from build123d import *

# Parameters (mm, degrees)
BOSS_EXTRUDE1_DEPTH   = 160
RIB3_REACH            = 111.505
SKETCH4_WALL_W        = 239.367706636
SKETCH4_WALL_H        = 3
RIB4_START            = -3
RIB4_DEPTH            = 3
F_6_CLEARANCE_HOLE1_D = 3.7973
SKETCH18_R            = 2.3495
CUT_EXTRUDE1_DEPTH    = 7.5
SKETCH19_R            = 2.6162
CUT_EXTRUDE2_DEPTH    = 6.35
SKETCH10_R            = 2.3495
CUT_EXTRUDE3_DEPTH    = 163.255727865
SKETCH20_R            = 2.6162
CUT_EXTRUDE4_DEPTH    = 6.35


# Read off the part's stored shape, not the designer's step: Rib4
with BuildPart() as part:
    # Sketch1 → Boss-Extrude1 (new body)
    with BuildSketch(Plane.XY):
        with BuildLine():
            Line((0, 0), (0, 12))
            Line((0, 12), (-8, 12))
            Line((-8, 12), (-8, 6))
            ThreePointArc((-8, 6), (-8.878679656, 3.878679656), (-11, 3))
            Line((-11, 3), (-24, 3))
            Line((-24, 3), (-24, 0))
            Line((-24, 0), (-8.5, 0))
            Line((-8.5, 0), (-8.5, -0.285))
            Line((-8.5, -0.285), (0, -0.285))
            Line((0, -0.285), (0, 0))
        make_face()
    extrude(amount=BOSS_EXTRUDE1_DEPTH)

    # Sketch4 wall → Rib3 (add, up to next)
    with BuildSketch(Plane(origin=(-16, 7.5, 53.83333334), x_dir=(-0.871575537125, -0.490261239633, 0), z_dir=(-0.490261239633, 0.871575537125, 0)), mode=Mode.PRIVATE) as rib3_sk1:
        Rectangle(SKETCH4_WALL_W, SKETCH4_WALL_H)
    rib3_tool1 = extrude(rib3_sk1.sketch, amount=-RIB3_REACH, mode=Mode.PRIVATE) - part.part
    rib3 = rib3_tool1.solids().sort_by_distance((-16, 7.5, 53.83333334))[0]
    add(rib3)

    # Rib4 outline → Rib4 (add)
    with BuildSketch(Plane(origin=(0, 0, 0), x_dir=(-1, 0, 0), z_dir=(0, 0, -1)).offset(RIB4_START)):
        with BuildLine():
            Line((24, 3), (8, 12))
            Line((8, 12), (8, 6))
            ThreePointArc((8, 6), (8.878679656, 3.878679656), (11, 3))
            Line((11, 3), (24, 3))
        make_face()
    rib4 = extrude(amount=RIB4_DEPTH)

    # Mirror1: Rib3, Rib4 across plane
    add(rib3.mirror(Plane(origin=(0, 0, 80), x_dir=(1, 0, 0), z_dir=(0, 0, -1))))
    add(rib4.mirror(Plane(origin=(0, 0, 80), x_dir=(1, 0, 0), z_dir=(0, 0, -1))))

    # 6 Clearance Hole1 (through all)
    with Locations(Plane(origin=(0, 0, 0), x_dir=(-1, 0, 0), z_dir=(0, -1, 0))):
        with Locations((17.49975, -10), (17.49975, -80), (17.49975, -150)):
            Hole(F_6_CLEARANCE_HOLE1_D / 2)

    # Sketch18 → Cut-Extrude1 (cut)
    with BuildSketch(Plane(origin=(0, 0, 0), x_dir=(0, 0, -1), z_dir=(1, 0, 0))):
        with Locations((-133.333333335, 5.8575)):
            Circle(SKETCH18_R)
        with Locations((-26.666666667, 5.8575)):
            Circle(SKETCH18_R)
        with Locations((-80, 5.8575)):
            Circle(SKETCH18_R)
    extrude(amount=-CUT_EXTRUDE1_DEPTH, mode=Mode.SUBTRACT)

    # Sketch19 → Cut-Extrude2 (cut)
    with BuildSketch(Plane(origin=(0, 0, 0), x_dir=(0, 0, -1), z_dir=(1, 0, 0))):
        with Locations((-133.333333335, 5.8575)):
            Circle(SKETCH19_R)
        with Locations((-26.666666667, 5.8575)):
            Circle(SKETCH19_R)
        with Locations((-80, 5.8575)):
            Circle(SKETCH19_R)
    extrude(amount=-CUT_EXTRUDE2_DEPTH, mode=Mode.SUBTRACT)

    # Sketch10 → Cut-Extrude3 (cut, through all)
    with BuildSketch(Plane(origin=(0, -0.285, 0), x_dir=(-1, 0, 0), z_dir=(0, -1, 0))):
        with Locations(Location((4.749875, -42.33333334, 0), (0, 0, 90))):
            Circle(SKETCH10_R)
        with Locations(Location((4.749875, -117.66666666, 0), (0, 0, 90))):
            Circle(SKETCH10_R)
    extrude(amount=-CUT_EXTRUDE3_DEPTH, mode=Mode.SUBTRACT)

    # Sketch20 → Cut-Extrude4 (cut)
    with BuildSketch(Plane.XZ.offset(0.285)):
        with Locations(Location((-4.749875, 117.66666666, 0), (0, 0, 270))):
            Circle(SKETCH20_R)
        with Locations(Location((-4.749875, 42.33333334, 0), (0, 0, 270))):
            Circle(SKETCH20_R)
    extrude(amount=-CUT_EXTRUDE4_DEPTH, mode=Mode.SUBTRACT)


solid = part.part
Part model, mm, in its own coordinate system. A direction names the side the tool comes from. Round coordinates to 2 decimals unless told otherwise and drop trailing zeros. Write each loop counter-clockwise with the first axis right and the second up, starting at its lowest first coordinate (ties: lowest second). Pieces come first, ordered by that corner, then holes. Notation, with made-up numbers: M 69,58 L 87,58 A34 cw 87,95 Z; hole C -22,78 d6. An arc over 180 degrees is marked long. Return JSON: item names as keys, results as strings. Group by question number.
(1) Saw through at C-C on z = 91. Write the cut outline in (x, y) (3 decimals).
(2) Two-plate mould, pull along Z, no slides. Class faces 5 (the face through (0, 9, 79)), 6 (the face through (-3.131, 6.643, 130.838)): +Z half, -Z half, draft (parallel to the pull), parting line (faces both ways), or undercut.
(3) Saw through at A-A on z = 150. Write the cut outline in (x, y) (3 decimals), then the cut area to 3 significant figures.
(4) Pin check, flat tips, straight feed: pin 1 Ø4 at (x, z) = (-14.5, 24) entering from -Y; pin 2 Ø4 at (x, z) = (-4.75, 42.33) entering from -Y; pin 3 Ø3 at (y, z) = (9.5, 27) entering from -X; pin 4 Ø3 at (y, z) = (5.86, 26.67) entering from -X. Stop position of each tip, or through.
(5) Which spindle directions (+Z, -Z, +X, -X, +Y, -Y) get a long thin tool onto all of the face, cutting with end or side? Do faces 1 (the face through (-13, 6, 55.333)), 2 (the face through (-6.917, 5.961, 29.014)), 3 (the face through (-16.48, 1.52, 8.4)), 4 (the face through (-15, 0, 79)). Say none if no direction does.
(6) Saw through at B-B on z = 134. Write the cut outline in (x, y) (3 decimals).
(7) Drill centre lines: probe 1 along Z at (x, y) = (-13.5, 6); probe 2 along X at (y, z) = (1.15, 80); probe 3 along Z at (x, y) = (-4.5, 1.75). Where is each one in solid material? Low to high.
Returned:
{
 "1": {"outline": "M -24,0 L -8.5,0 L -8.5,-0.285 L 0,-0.285 L 0,12 L -8,12 L -8,6 A3 cw -11,3 L -24,3 Z"},
 "2": {"face 5": "draft", "face 6": "undercut"},
 "3": {"outline": "M -24,0 L -19.398,0 L -19.398,3 L -24,3 Z; M -15.601,0 L -8.5,0 L -8.5,-0.285 L 0,-0.285 L 0,12 L -8,12 L -8,6 A3 cw -11,3 L -15.601,3 Z", "area": "137 mm²"},
 "4": {"pin 1": "y = 0", "pin 2": "through", "pin 3": "x = -8", "pin 4": "x = -8.49"},
 "5": {"face 1": "-X, +Y", "face 2": "+X", "face 3": "+Y, -Y", "face 4": "+Z, -Z, -X, -Y"},
 "6": {"outline": "M -24,0 L -8.5,0 L -8.5,-0.285 L 0,-0.285 L 0,3.328 L -6.35,3.328 L -6.35,3.605 L -7.5,3.605 L -7.5,8.11 L -6.35,8.11 L -6.35,8.387 L 0,8.387 L 0,12 L -8,12 L -8,6 A3 cw -11,3 L -24,3 Z"},
 "7": {"probe 1": "0 to 3, 52.33 to 55.33, 104.67 to 107.67, 157 to 160", "probe 2": "-24 to -19.4, -15.6 to 0", "probe 3": "0 to 39.73, 44.94 to 115.06, 120.27 to 160"}
}
